Geometry check sheet. Reference: drawing and pictorial views, mm from the part's lowest x, y, z. A direction names the side the tool comes from. Give positions to 0.01 mm unless a question says otherwise; leave off trailing zeros. Write each loop counter-clockwise with the first axis right and the second up, starting at its lowest first coordinate (ties: lowest second). Pieces come first, ordered by that corner, then holes. Notation, with made-up numbers: M 21.25,15 L 40.25,15 A12 ccw 40.25,27 Z; hole C 77.25,-6 d8. An arc over 180 degrees is marked long. Answer as a JSON object with one key per item and string values.
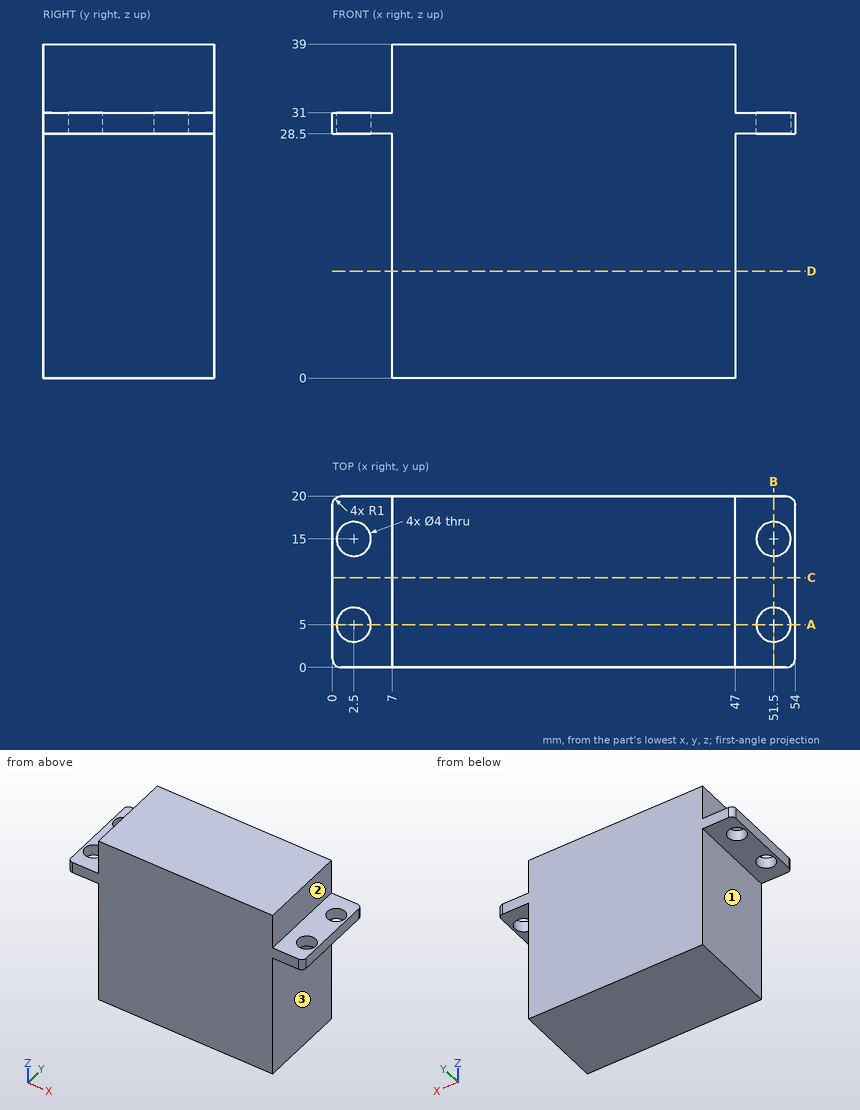
1) Access from +Z, -Z, +X, -X, +Y, -Y to the whole of each face (thin tool, end or side, straight path). Record for the marked faces 1, 2 and 3.
Completed:
{"face 1": "-Z, -X, +Y, -Y", "face 2": "+Z, +X, +Y, -Y", "face 3": "-Z, +X, +Y, -Y"}
2) Section check D-D on z = 12.5. Record the boundary of the cut face in (x, y).
Completed:
{"outline": "M 7,0 L 47,0 L 47,20 L 7,20 Z"}
3) Section check B-B on x = 51.5. Record the boundary of the cut face in (y, z), and give its area (3 significant figures).
Completed:
{"outline": "M 0,28.5 L 3,28.5 L 3,31 L 0,31 Z; M 7,28.5 L 13,28.5 L 13,31 L 7,31 Z; M 17,28.5 L 20,28.5 L 20,31 L 17,31 Z", "area": "30.0 mm2"}
4) Thickness scan on L1, parallel to Y at x = 2.5, z = 29.4; L2, parallel to Y at x = 2, z = 29; L3, parallel to X at y = 13, z = 34.5. Record the ranges inside material, lowest first.
Completed:
{"L1": "y = 0 to 3, 7 to 13, 17 to 20", "L2": "y = 0 to 3.06, 6.94 to 13.06, 16.94 to 20", "L3": "x = 7 to 47"}
5) Go/stop test with flat-tipped pins: pin 1 (2 mm diameter, centred on x = 49, y = 8.5, fed in from +Z); pin 2 (6 mm diameter, centred on y = 7.5, z = 4, fed in from -X); pin 3 (9 mm diameter, centred on y = 9.5, z = 34, fed in from -X); pin 4 (2.5 mm diameter, centred on x = 2.5, y = 5, fed in from -Z). Record where each tip stops, or that it passes through.
Completed:
{"pin 1": "stops at z = 31", "pin 2": "stops at x = 7", "pin 3": "stops at x = 0", "pin 4": "passes through"}
6) Section check A-A on y = 5. Record the boundary of the cut face in (x, z), and give its area (4 significant figures).
Completed:
{"outline": "M 0,28.5 L 0.5,28.5 L 0.5,31 L 0,31 Z; M 4.5,28.5 L 7,28.5 L 7,0 L 47,0 L 47,28.5 L 49.5,28.5 L 49.5,31 L 47,31 L 47,39 L 7,39 L 7,31 L 4.5,31 Z; M 53.5,28.5 L 54,28.5 L 54,31 L 53.5,31 Z", "area": "1,575 mm2"}
7) Section check C-C on y = 10.5. Record the boundary of the cut face in (x, z), and give its area (4 significant figures).
Completed:
{"outline": "M 0,28.5 L 7,28.5 L 7,0 L 47,0 L 47,28.5 L 54,28.5 L 54,31 L 47,31 L 47,39 L 7,39 L 7,31 L 0,31 Z", "area": "1,595 mm2"}
